from build123d import *

# Parameters (mm, degrees)
BOSS_EXTRUDE1_DEPTH = 10


with BuildPart() as part:
    # Sketch1 → Boss-Extrude1 (new body)
    with BuildSketch(Plane(origin=(0, 0, 0), x_dir=(1, 0, 0), z_dir=(0, 1, 0))):
        Polygon((-222.25, -751.824242644), (-222.25, -802.624242644), (-232.25, -802.624242644), (-232.25, -853.424242644), (-222.25, -853.424242644), (-222.25, -904.224242644), (-232.25, -904.224242644), (-232.25, -955.024242644), (-222.25, -955.024242644), (-222.25, -1005.824242644), (222.25, -1005.824242644), (222.25, -955.024242644), (232.25, -955.024242644), (232.25, -904.224242644), (222.25, -904.224242644), (222.25, -853.424242644), (232.25, -853.424242644), (232.25, -802.624242644), (222.25, -802.624242644), (222.25, -751.824242644), (223.558028711, -725.663668424), (233.5455521, -726.163044593), (236.082383041, -675.426425778), (226.094859652, -674.927049609), (228.631690593, -624.190430794), (238.619213981, -624.689806963), (241.156044922, -573.953188148), (231.168521533, -573.453811979), (233.705352474, -522.717193164), (243.692875863, -523.216569333), (246.229706804, -472.479950518), (236.242183415, -471.980574349), (238.779014356, -421.243955534), (248.766537744, -421.743331703), (251.303368685, -371.006712888), (241.315845296, -370.507336719), (243.852676237, -319.770717904), (253.840199626, -320.270094073), (256.377030567, -269.533475258), (246.389507178, -269.034099089), (248.926338119, -218.297480274), (258.913861507, -218.796856443), (261.450692448, -168.060237628), (251.463169059, -167.560861459), (254, -116.824242644), (117.602, -33.957645835), (95.25, 111.775757356), (-95.25, 111.775757356), (-117.475, -33.759249998), (-254, -116.824242644), (-251.463169059, -167.560861459), (-261.450692448, -168.060237628), (-258.913861507, -218.796856443), (-248.926338119, -218.297480274), (-246.389507178, -269.034099089), (-256.377030567, -269.533475258), (-253.840199626, -320.270094073), (-243.852676237, -319.770717904), (-241.315845296, -370.507336719), (-251.303368685, -371.006712888), (-248.766537744, -421.743331703), (-238.779014356, -421.243955534), (-236.242183415, -471.980574349), (-246.229706804, -472.479950518), (-243.692875863, -523.216569333), (-233.705352474, -522.717193164), (-231.168521533, -573.453811979), (-241.156044922, -573.953188148), (-238.619213981, -624.689806963), (-228.631690593, -624.190430794), (-226.094859652, -674.927049609), (-236.082383041, -675.426425778), (-233.5455521, -726.163044593), (-223.558028711, -725.663668424), align=None)
    extrude(amount=BOSS_EXTRUDE1_DEPTH)


solid = part.part
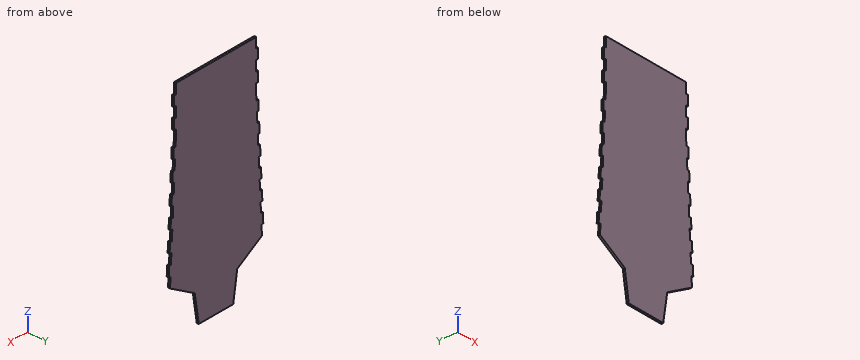
Input: part model. Units: mm. Frame: model coordinates. Coordinates: 2 decimals unless noted, no trailing zeros. Order: outer loops, then holes, each group sorted by start corner. A loop starts at its lowest first (then second) coordinate and runs counter-clockwise, first axis right, second up. Notation, with made-up numbers: M 27,54.25 L 46,54.25 A5 cw 46,63.25 Z; hole C -38.75,-27.5 d8. An arc over 180 degrees is marked long. Answer in a Markdown table with one row per item.
(1) Section query B-B, the plane z = 598.5. Output: boundary loops of the cut face in (x, y).
Numbers:
| item | result |
|---|---|
| outline | M -239.93,0 L 239.93,0 L 239.93,10 L -239.93,10 Z |
(2) Material intervals for line 1 (X direction, y = 2.75, z = 912); line 2 (X direction, y = 9, z = 870); line 3 (Z direction, x = -194.5, y = 7), sorted ascending. Write a range as [from, to].
Numbers:
| item | result |
|---|---|
| line 1 | x = [-232.25, 232.25] |
| line 2 | x = [-222.25, 222.25] |
| line 3 | z = [80.62, 1005.82] |
(3) Section query A-A, the plane x = 151.5. Output: boundary loops of the cut face in (y, z), plus the area to 3 significant figures.
Numbers:
| item | result |
|---|---|
| outline | M 0,54.55 L 10,54.55 L 10,1005.82 L 0,1005.82 Z |
| area | 9,510 mm^2 |
(4) Contact query for flat-ended pins moving along their axis: pin 1 Ø4 at (y, z) = (3, 541) entering from -X; pin 2 Ø4 at (y, z) = (3, 246) entering from +X; pin 3 Ø3 at (x, y) = (-226.5, 6) entering from +Z. Output: stop coordinate, or through.
Numbers:
| item | result |
|---|---|
| pin 1 | stops at x = -232.89 |
| pin 2 | stops at x = 247.64 |
| pin 3 | stops at z = 955.02 |
